```python
from build123d import *

# Parameters (mm, degrees)
BOSS_EXTRUDE1_DEPTH = 28
BOSS_EXTRUDE2_DEPTH = 5
BOSS_EXTRUDE6_START = 40
BOSS_EXTRUDE6_DEPTH = 40


with BuildPart() as part:
    # Sketch1 → Boss-Extrude1 (new body)
    with BuildSketch(Plane.XY):
        Polygon((10.849101299, 4.6), (12.849101299, 2.6), (17.349101299, 2.6), (17.349101299, 17.249101299), (-37.349101299, 17.249101299), (-37.349101299, -17.249101299), (17.349101299, -17.249101299), (17.349101299, -2.6), (12.849101299, -2.6), (10.849101299, -4.6), (10.849101299, -10.749101299), (-30.849101299, -10.749101299), (-30.849101299, 10.749101299), (10.849101299, 10.749101299), align=None)
    extrude(amount=-BOSS_EXTRUDE1_DEPTH)

    # Sketch2 → Boss-Extrude2 (add)
    with BuildSketch(Plane(origin=(0, 0, -28), x_dir=(-1, 0, 0), z_dir=(0, 0, -1))):
        with BuildLine():
            Line((-12.849101299, 2.6), (-41.057604209, 2.6))
            ThreePointArc((-41.057604209, 2.6), (41.139845204, 0), (-41.057604209, -2.6))
            Line((-41.057604209, -2.6), (-12.849101299, -2.6))
            Line((-12.849101299, -2.6), (-12.849101299, 2.6))
        make_face()
    extrude(amount=BOSS_EXTRUDE2_DEPTH)

    # Sketch3 → Boss-Extrude6 (add)
    with BuildSketch(Plane.XY.offset(-28).offset(BOSS_EXTRUDE6_START)):
        with BuildLine():
            Line((-37.349101299, 17.249101299), (17.349101299, 17.249101299))
            Line((17.349101299, 17.249101299), (17.349101299, 2.6))
            Line((17.349101299, 2.6), (41.057604209, 2.6))
            ThreePointArc((41.057604209, 2.6), (7.55561319, 40.440073847), (-37.349101299, 17.249101299))
        make_face()
        with BuildLine():
            Line((41.057604209, -2.6), (17.349101299, -2.6))
            Line((17.349101299, -2.6), (17.349101299, -17.249101299))
            Line((17.349101299, -17.249101299), (-37.349101299, -17.249101299))
            ThreePointArc((-37.349101299, -17.249101299), (7.55561319, -40.440073847), (41.057604209, -2.6))
        make_face()
    extrude(amount=-BOSS_EXTRUDE6_DEPTH)


solid = part.part
```
Verification items for the finished model (mm, model axes). A direction names the side the tool comes from. Round coordinates to 2 decimals unless told otherwise and drop trailing zeros. Write each loop counter-clockwise with the first axis right and the second up, starting at its lowest first coordinate (ties: lowest second). Pieces come first, ordered by that corner, then holes. Notation, with made-up numbers: (-10.5, 12.5) - (0.5, 12.5) arc R20 cw to (0.5, 30.5) - close; hole circle Ø3 at (-13.5, 19.5). An arc over 180 degrees is marked (long way). Answer as a JSON object with one key per item and string values. Group by question number.
Q1. Section check D-D, the plane x = 0. Enter the section's corners in (y, z), plus the area to 3 significant figures.
Q2. Section check B-B, the plane y = 0. Enter the section's corners in (x, z), plus the area to 3 significant figures.
Q3. Mould release check, pull along X, two halves, no side actions. Record for faces 1 (the flat face through (-37.349, 0, -14)), 2 (the flat face through (-10, -10.749, -14)), 3 (the flat face through (10.849, 8, -14)), 4 (the flat face through (1, 22, 12)): released by +X, released by -X, zero draft, split by the parting line, or undercut.
Q4. Thickness scan on line 1 (X direction, y = 7.5, z = -9.5); line 2 (Y direction, x = 20, z = -18.5); line 3 (X direction, y = 5, z = -8.5). Record the ranges inside material, lowest first.
Q5. Go/stop test with flat-tipped pins: pin 1 Ø3.5 at (x, z) = (-19.5, 5) entering from +Y; pin 2 Ø13 at (y, z) = (-10.5, 3) entering from -X; pin 3 Ø4 at (x, y) = (-39, -3) entering from +Z. Record where each tip stops, or that it passes through.
Q6. Section check C-C, the plane z = -2. Enter the section's corners in (x, y), plus the area to 3 significant figures.
Q7. Tool access check on faces 5 (the flat face through (-10, -17.249, 6)), 6 (the flat face through (11.84, 3.61, -13.8)), 7 (the flat face through (12.849, 0, -30)). Record the directions out of +Z, -Z, +X, -X, +Y, -Y that give a thin tool (end or side, any length) a straight path to the whole face; none if there is none.
Q8. Section check A-A, the plane z = 8. Enter the section's corners in (x, y), plus the area to 3 significant figures.
Found:
{
 "1": {"outline": "(-41.14, -33) - (41.14, -33) - (41.14, 12) - (17.25, 12) - (17.25, 0) - (10.75, 0) - (10.75, -28) - (-10.75, -28) - (-10.75, 0) - (-17.25, 0) - (-17.25, 12) - (-41.14, 12) - close", "area": "2,690 mm^2"},
 "2": {"outline": "(-41.14, -33) - (12.85, -33) - (12.85, -28) - (-30.85, -28) - (-30.85, 0) - (-37.35, 0) - (-37.35, -28) - (-41.14, -28) - close", "area": "452 mm^2"},
 "3": {"face 1": "released by -X", "face 2": "undercut", "face 3": "undercut", "face 4": "zero draft"},
 "4": {"line 1": "x = -37.35 to -30.85, 10.85 to 40.45", "line 2": "y = -35.95 to -2.6, 2.6 to 35.95", "line 3": "x = -37.35 to -30.85, 10.85 to 40.83"},
 "5": {"pin 1": "stops at y = 37.11", "pin 2": "stops at x = -37.35", "pin 3": "stops at z = 0"},
 "6": {"outline": "(-37.35, -17.25) arc R41.14 ccw to (41.06, -2.6) - (12.85, -2.6) - (10.85, -4.6) - (10.85, -10.75) - (-30.85, -10.75) - (-30.85, 10.75) - (10.85, 10.75) - (10.85, 4.6) - (12.85, 2.6) - (41.06, 2.6) arc R41.14 ccw to (-37.35, 17.25) - close", "area": "4,170 mm^2"},
 "7": {"face 5": "+Z, -X", "face 6": "+Z", "face 7": "+Z, -Z, +X"},
 "8": {"outline": "(-37.35, -17.25) arc R41.14 ccw to (41.06, -2.6) - (17.35, -2.6) - (17.35, -17.25) - close; (-37.35, 17.25) - (17.35, 17.25) - (17.35, 2.6) - (41.06, 2.6) arc R41.14 ccw to start", "area": "3,220 mm^2"}
}
